Model file for the job. Use its own axes, mm. Round coordinates to 2 decimals unless told otherwise and drop trailing zeros. Order: outer loops, then holes, each group sorted by start corner. A loop starts at its lowest first (then second) coordinate and runs counter-clockwise, first axis right, second up. Notation, with made-up numbers: (6.5, 30.25) - (52.5, 30.25) arc R29 cw to (52.5, 54.25) - close; hole circle Ø7 at (51.5, 58). An arc over 180 degrees is marked (long way). Use one line per item in the form item = value.
from build123d import *

# Parameters (mm, degrees)
SKETCH2_R           = 35
BOSS_EXTRUDE1_DEPTH = 1.5
FILLET1_R           = 5


with BuildPart() as part:
    # Sketch1 → Revolve1 (revolve)
    with BuildSketch(Plane.XY):
        Polygon((35, 53.703703704), (44, -62.296296296), (42.62962963, -62.296296296), (33.5, 53.703703704), align=None)
    revolve(axis=Axis((0, 53.703703704, 0), (0, -1, 0)))

    # Sketch2 → Boss-Extrude1 (add)
    with BuildSketch(Plane(origin=(0, 53.703703704, 0), x_dir=(1, 0, 0), z_dir=(0, 1, 0))):
        Circle(SKETCH2_R)
    extrude(amount=-BOSS_EXTRUDE1_DEPTH)

    # Fillet1
    fillet1_edges = [part.edges().sort_by_distance(p)[0] for p in [
        (-33.618055556, 52.203703704, 0),
    ]]
    fillet(fillet1_edges, radius=FILLET1_R)


solid = part.part
(1) Pin check, flat tips, straight feed: pin 1 (4 mm diameter, centred on y = -43.5, z = 11, fed in from -X); pin 2 (4 mm diameter, centred on y = -29, z = 34.5, fed in from -X); pin 3 (10 mm diameter, centred on x = -12.5, z = 2.5, fed in from -Y). Stop position of each tip, or through.
Report:
pin_1 = -41.61
pin_2 = -25.69
pin_3 = 52.2
(2) Slice it at A-A on x = 0. Give the cut face in (y, z), then the cut area to 3 significant figures.
Report:
outline = (-62.3, -44) - (53.7, -35) - (53.7, 35) - (-62.3, 44) - (-62.3, 42.63) - (47.6, 33.98) arc R5 cw to (52.2, 29) - (52.2, -29) arc R5 cw to (47.6, -33.98) - (-62.3, -42.63) - close
area = 443 mm2
(3) Probe probe 1 along Z at (x, y) = (-6.5, -46.5); probe 2 along Z at (x, y) = (-26, 23); probe 3 along Y at (x, z) = (7.5, 27). List the from-to ranges inside material, lowest first. Write a range as [from, to].
Report:
probe_1 = [-42.28, -40.87], [40.87, 42.28]
probe_2 = [-26.86, -24.78], [24.78, 26.86]
probe_3 = [52.2, 53.7]
(4) Slice it at B-B on z = 0. Give the cut face in (x, y).
Report:
outline = (-44, -62.3) - (-42.63, -62.3) - (-33.98, 47.6) arc R5 cw to (-29, 52.2) - (29, 52.2) arc R5 cw to (33.98, 47.6) - (42.63, -62.3) - (44, -62.3) - (35, 53.7) - (-35, 53.7) - close
(5) Pull direction Z, two halves, no side cores. Call faces 1 (the face through (-36.1, -62.296, 23)), 2 (the face through (0, 52.204, 0)), 3 (the face through (37.736, -5.108, 11.884)): released by +Z, released by -Z, zero draft, split by the parting line, or undercut.
Report:
face_1 = zero draft
face_2 = undercut
face_3 = split by the parting line
(6) Slice it at C-C on y = 29.5. Give the cut face in (x, z), then the cut area to 3 significant figures.
Report:
outline = circle Ø73.76 at (0, 0); hole circle Ø70.81 at (0, 0)
area = 334 mm2
(7) Slice it at D-D on y = 41.5. Give the cut face in (x, z), then the cut area to 3 significant figures.
Report:
outline = circle Ø71.89 at (0, 0); hole circle Ø68.92 at (0, 0)
area = 329 mm2
